from build123d import *

# Parameters (mm, degrees)
BOSS_EXTRUDE1_DEPTH            = 28.575
HOLE1_D                        = 6.35
HOLE1_DEPTH                    = 12.7
HOLE1_CBORE_D                  = 12.7
HOLE1_CBORE_DEPTH              = 3.175
HOLE1_TIP                      = 1.907732465
F_5_16_0_3125_DIAMETER_HOLE1_D = 7.9375


with BuildPart() as part:
    # Sketch1 → Boss-Extrude1 (new body)
    with BuildSketch(Plane(origin=(0, 0, 0), x_dir=(1, 0, 0), z_dir=(0, 1, 0))):
        Polygon((-52.3875, 0), (52.3875, 0), (52.3875, -12.7), (28.575, -12.7), (28.575, -6.35), (-28.575, -6.35), (-28.575, -12.7), (-52.3875, -12.7), align=None)
    extrude(amount=BOSS_EXTRUDE1_DEPTH)

    # Hole1
    with Locations(Plane(origin=(0, 0, 0), x_dir=(-1, 0, 0), z_dir=(0, 0, -1))):
        with Locations((-12.7, 14.2875), (12.7, 14.2875)):
            CounterBoreHole(HOLE1_D / 2, HOLE1_CBORE_D / 2, HOLE1_CBORE_DEPTH, depth=HOLE1_DEPTH)
            with Locations((0, 0, -(HOLE1_DEPTH + HOLE1_TIP / 2))):  # 118° drill point
                Cone(0, HOLE1_D / 2, HOLE1_TIP, mode=Mode.SUBTRACT)

    # 5/16 (0.3125) Diameter Hole1 (through all)
    with Locations(Plane.XY.offset(12.7)):
        with Locations((-39.6875, 14.2875), (39.6875, 14.2875)):
            Hole(F_5_16_0_3125_DIAMETER_HOLE1_D / 2)


solid = part.part
Model file for the job. Use its own axes, mm. A direction names the side the tool comes from. Give positions to 0.01 mm unless a question says otherwise; leave off trailing zeros. Loops run counter-clockwise (first coordinate to the right, second up) from the corner with the lowest first, then second, coordinate; pieces in that order, holes last.
1) Wall check: line 1 (Y direction, x = -13, z = 5.5) (3 decimals); line 2 (Y direction, x = 12.7, z = 4.3) (1 decimal); line 3 (X direction, y = 18.75, z = 10.5) (1 decimal). Give the ranges that are in metal, low to high.
2) Tool access for faces 4 (the flat face through (-28.575, 14, 9)), 5 (the flat face through (-15.4, 11.6, 3.175)), 6 (the flat face through (1, 0, 5)): list every direction of +Z, -Z, +X, -X, +Y, -Y with a clear straight run to the whole face (end or side of a thin tool).
3) Pull direction X, two halves, no side cores. Call faces 1 (the cylindrical face through (-36.54, 11.87, 6.26)), 2 (the flat face through (52.388, 14, 6)), 3 (the flat face through (-1, 14, 0)): +X half, -X half, draft (parallel to the pull), parting line (faces both ways), or undercut.
4) Flat gauge pins, fed straight in: pin 1 Ø8.5 at (x, y) = (-12.7, 14.29) entering from +Z; pin 2 Ø10 at (x, y) = (12.7, 14.29) entering from -Z (3 decimals). Where does each tip first touch, or does it go through?
5) Saw through at B-B (z = 9.75). Write the cut outline in (x, y) (1 decimal), plus the area to 3 significant figures.
6) Saw through at D-D (x = -40.5). Write the cut outline in (y, z) (3 decimals).
Answer block:
1. line 1: y = 0 to 11.127, 17.448 to 28.575
1. line 2: y = 0 to 11.1, 17.5 to 28.6
1. line 3: x = -52.4 to -28.6, 28.6 to 52.4
2. face 4: +Z, +Y, -Y
2. face 5: -Z
2. face 6: +Z, -Z, +X, -X, -Y
3. face 1: undercut
3. face 2: +X half
3. face 3: draft
4. pin 1: stops at z = 6.35
4. pin 2: stops at z = 3.175
5. outline: (-52.4, 0) - (-28.6, 0) - (-28.6, 28.6) - (-52.4, 28.6) - close; (28.6, 0) - (52.4, 0) - (52.4, 28.6) - (28.6, 28.6) - close; hole circle Ø7.9 at (-39.7, 14.3); hole circle Ø7.9 at (39.7, 14.3)
5. area: 1,260 mm2
6. outline: (0, 0) - (10.403, 0) - (10.403, 12.7) - (0, 12.7) - close; (18.172, 0) - (28.575, 0) - (28.575, 12.7) - (18.172, 12.7) - close
